```python
from build123d import *

# Parameters (mm, degrees)
SKETCH1_R           = 2.1463
BOSS_EXTRUDE1_DEPTH = 1.5748


with BuildPart() as part:
    # Sketch1 → Boss-Extrude1 (new body)
    with BuildSketch(Plane.XY.offset(1.5748)):
        Polygon((6.35, 34.284985055), (6.35, 43.3324), (4.7244, 44.958), (-3.9116, 44.958), (-5.5372, 43.3324), (-5.5372, 34.284985055), (-3.891214945, 32.639), (-5.5372, 30.993014945), (-5.5372, 21.584985055), (-3.891214945, 19.939), (-5.5372, 18.293014945), (-5.5372, 4.313373781), (4.313373781, -5.5372), (18.293014945, -5.5372), (19.939, -3.891214945), (21.584985055, -5.5372), (30.993014945, -5.5372), (32.639, -3.891214945), (34.284985055, -5.5372), (43.3324, -5.5372), (44.958, -3.9116), (44.958, 4.7244), (43.3324, 6.35), (34.284985055, 6.35), (32.639, 4.704014945), (30.993014945, 6.35), (21.584985055, 6.35), (19.939, 4.704014945), (18.293014945, 6.35), (12.7, 6.35), (6.35, 12.7), (6.35, 18.293014945), (4.704014945, 19.939), (6.35, 21.584985055), (6.35, 30.993014945), (4.704014945, 32.639), align=None)
        with Locations((2.828780678, 2.828780678)):
            Circle(SKETCH1_R, mode=Mode.SUBTRACT)
        with BuildLine():
            Line((12.7, 2.0955), (14.478, 2.0955))
            ThreePointArc((14.478, 2.0955), (16.5735, 0), (14.478, -2.0955))
            Line((14.478, -2.0955), (12.7, -2.0955))
            ThreePointArc((12.7, -2.0955), (10.6045, 0), (12.7, 2.0955))
        make_face(mode=Mode.SUBTRACT)
        with BuildLine():
            Line((-2.0955, 38.1), (-2.0955, 39.878))
            ThreePointArc((-2.0955, 39.878), (0, 41.9735), (2.0955, 39.878))
            Line((2.0955, 39.878), (2.0955, 38.1))
            ThreePointArc((2.0955, 38.1), (0, 36.0045), (-2.0955, 38.1))
        make_face(mode=Mode.SUBTRACT)
        with BuildLine():
            Line((-2.0955, 12.7), (-2.0955, 14.478))
            ThreePointArc((-2.0955, 14.478), (0, 16.5735), (2.0955, 14.478))
            Line((2.0955, 14.478), (2.0955, 12.7))
            ThreePointArc((2.0955, 12.7), (0, 10.6045), (-2.0955, 12.7))
        make_face(mode=Mode.SUBTRACT)
        with BuildLine():
            Line((-2.0955, 25.4), (-2.0955, 27.178))
            ThreePointArc((-2.0955, 27.178), (0, 29.2735), (2.0955, 27.178))
            Line((2.0955, 27.178), (2.0955, 25.4))
            ThreePointArc((2.0955, 25.4), (0, 23.3045), (-2.0955, 25.4))
        make_face(mode=Mode.SUBTRACT)
        with BuildLine():
            Line((25.4, 2.0955), (27.178, 2.0955))
            ThreePointArc((27.178, 2.0955), (29.2735, 0), (27.178, -2.0955))
            Line((27.178, -2.0955), (25.4, -2.0955))
            ThreePointArc((25.4, -2.0955), (23.3045, 0), (25.4, 2.0955))
        make_face(mode=Mode.SUBTRACT)
        with BuildLine():
            Line((38.1, 2.0955), (39.878, 2.0955))
            ThreePointArc((39.878, 2.0955), (41.9735, 0), (39.878, -2.0955))
            Line((39.878, -2.0955), (38.1, -2.0955))
            ThreePointArc((38.1, -2.0955), (36.0045, 0), (38.1, 2.0955))
        make_face(mode=Mode.SUBTRACT)
    extrude(amount=-BOSS_EXTRUDE1_DEPTH)


solid = part.part
```
Verification items for the finished model (mm, model axes). A direction names the side the tool comes from. Round coordinates to 2 decimals unless told otherwise and drop trailing zeros. Order: outer loops, then holes, each group sorted by start corner. A loop starts at its lowest first (then second) coordinate and runs counter-clockwise, first axis right, second up. Notation, with made-up numbers: (4, 47.25) -> (35, 47.25) arc R9 cw to (35, 55.25) -> close; hole circle Ø9 at (30, 67.5). An arc over 180 degrees is marked (long way). Put each result on its own line as item: value. Start each with the question number.
(1) Draft check along X on faces 1 (the face through (11, -5.537, 1)), 2 (the face through (0.046, 10.605, 0.798)), 3 (the face through (-5.537, 11, 1)). Enter one of: +X half, -X half, draft (parallel to the pull), parting line (faces both ways), or undercut.
(2) Depth check by flat-ended pin: pin 1 Ø0.5 at (x, z) = (24.5, 1) entering from +Y; pin 2 Ø8 at (x, y) = (6, 33) entering from -Z; pin 3 Ø0.5 at (y, z) = (26.5, 0.5) entering from +X. Enter the tip coordinate at first touch or a pass-through.
(3) Material ranges on line 1 along Y through (x, z) = (27, 0.6); line 2 along Y through (x, z) = (5.5, 0.2), recorded low to high.
(4) Section check B-B (y = 0). Enter the section's corners in (x, z).
(5) Section check C-C (y = 16). Enter the section's corners in (x, z).
(6) Section check A-A (x = 13.5). Enter the section's corners in (y, z), then the cut area to 3 significant figures.
(7) Tool access check on faces 4 (the face through (19.1, -4.73, 0.8)), 5 (the face through (-0.046, 16.573, 0.798)), 6 (the face through (16, 6.35, 1)). Record the directions out of +Z, -Z, +X, -X, +Y, -Y that give a thin tool (end or side, any length) a straight path to the whole face; none if there is none.
Completed:
1. face 1: draft
1. face 2: undercut
1. face 3: -X half
2. pin 1: stops at y = 6.35
2. pin 2: stops at z = 0
2. pin 3: stops at x = 6.35
3. line 1: y = -5.54 to -2.1, 2.1 to 6.35
3. line 2: y = -5.54 to 19.14, 20.73 to 31.84, 33.43 to 44.18
4. outline: (-1.22, 0) -> (10.6, 0) -> (10.6, 1.57) -> (-1.22, 1.57) -> close; (16.57, 0) -> (23.3, 0) -> (23.3, 1.57) -> (16.57, 1.57) -> close; (29.27, 0) -> (36, 0) -> (36, 1.57) -> (29.27, 1.57) -> close; (41.97, 0) -> (44.96, 0) -> (44.96, 1.57) -> (41.97, 1.57) -> close
5. outline: (-5.54, 0) -> (-1.44, 0) -> (-1.44, 1.57) -> (-5.54, 1.57) -> close; (1.44, 0) -> (6.35, 0) -> (6.35, 1.57) -> (1.44, 1.57) -> close
6. outline: (-5.54, 0) -> (-2.1, 0) -> (-2.1, 1.57) -> (-5.54, 1.57) -> close; (2.1, 0) -> (6.35, 0) -> (6.35, 1.57) -> (2.1, 1.57) -> close
6. area: 12.1 mm2
7. face 4: +Z, -Z, -Y
7. face 5: +Z, -Z
7. face 6: +Z, -Z, +X, +Y
